Check sheet for the modelled part. Datum: model origin and axes. Units: mm. Face numbers are marked on the shaded views. A direction names the side the tool comes from. Coordinates: 2 decimals unless noted, no trailing zeros. Order: outer loops, then holes, each group sorted by start corner. A loop starts at its lowest first (then second) coordinate and runs counter-clockwise, first axis right, second up.
1. Set-up check for the marked faces 1, 2 and 3: record each of +Z, -Z, +X, -X, +Y, -Y from which the full face is reachable in a straight line by a thin tool's end or side.
2. Cross-section at A-A (y = 0). Enter the section's corners in (x, z), then the cut area to 3 significant figures.
3. Gauge pin test, flat ends, axial feed: pin 1 Ø16 at (y, z) = (5.5, 36.5) entering from +X; pin 2 Ø6.5 at (y, z) = (0, 13.5) entering from +X; pin 3 Ø3 at (y, z) = (-0.5, 14.5) entering from +X; pin 4 Ø4 at (x, y) = (18.5, -11.5) entering from -Z. Record the tip position at first contact, or that the pin passes through.
4. Cross-section at B-B (x = 11.25). Enter the section's corners in (y, z), then the cut area to 3 significant figures.
5. Draft check along Z on the marked faces 4, 5, 6 and 7. Enter one of: released by +Z, released by -Z, zero draft, split by the parting line, or undercut.
6. Thickness scan on line 1 (Y direction, x = 0.45, z = 36.5); line 2 (Y direction, x = -0.85, z = 36.5); line 3 (X direction, y = -7, z = 4). Record the ranges inside material, lowest first.
7. Cross-section at D-D (x = 3). Enter the section's corners in (y, z), then the cut area to 3 significant figures.
8. Cross-section at C-C (z = 13.5). Enter the section's corners in (x, y), then the cut area to 4 significant figures.
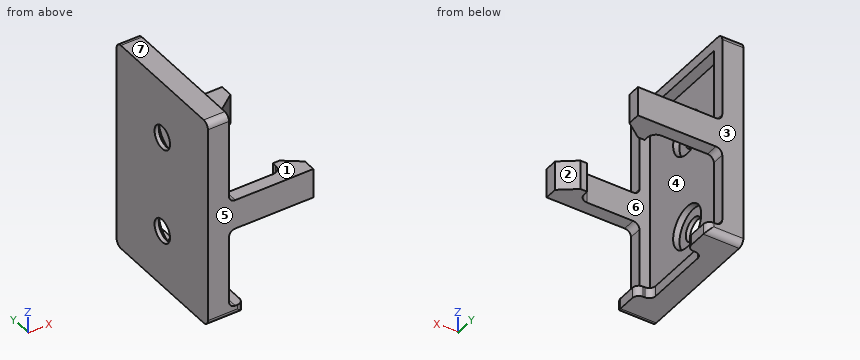
```python
from build123d import *

# Parameters (mm, degrees)
SKETCH1_W           = 2.5
SKETCH1_H           = 32.5
BOSS_EXTRUDE1_DEPTH = 50
SKETCH5_R           = 2.75
CUT_EXTRUDE5_DEPTH  = 30.5
SKETCH6_R           = 5
CUT_EXTRUDE6_DEPTH  = 1.5
SKETCH7_W           = 50
SKETCH7_H           = 32.5
SKETCH7_W_2         = 45
SKETCH7_H_2         = 26.5
BOSS_EXTRUDE2_DEPTH = 2.5
SKETCH8_W           = 7
SKETCH8_H           = 6
BOSS_EXTRUDE3_DEPTH = 20
CUT_EXTRUDE9_DEPTH  = 20
SKETCH10_W          = 3.5
SKETCH10_H          = 7.25
BOSS_EXTRUDE4_DEPTH = 2.5
FILLET1_R           = 1.5


with BuildPart() as part:
    # Sketch1 → Boss-Extrude1 (new body)
    with BuildSketch(Plane.XY):
        Rectangle(SKETCH1_W, SKETCH1_H)
    extrude(amount=BOSS_EXTRUDE1_DEPTH)

    # Sketch5 → Cut-Extrude5 (cut)
    with BuildSketch(Plane.ZY.offset(1.25)):
        with Locations((13.5, 0)):
            Circle(SKETCH5_R)
        with Locations((36.5, 0)):
            Circle(SKETCH5_R)
    extrude(amount=-CUT_EXTRUDE5_DEPTH, mode=Mode.SUBTRACT)

    # Sketch6 → Cut-Extrude6 (cut)
    with BuildSketch(Plane(origin=(1.25, 0, 0), x_dir=(0, 0, -1), z_dir=(1, 0, 0))):
        with Locations((-36.5, 0)):
            Circle(SKETCH6_R)
        with Locations((-13.5, 0)):
            Circle(SKETCH6_R)
    extrude(amount=-CUT_EXTRUDE6_DEPTH, mode=Mode.SUBTRACT)

    # Sketch7 → Boss-Extrude2 (add)
    with BuildSketch(Plane(origin=(1.25, 0, 0), x_dir=(0, 0, -1), z_dir=(1, 0, 0))):
        with Locations((-25, 0)):
            Rectangle(SKETCH7_W, SKETCH7_H)
        with Locations((-25, 0)):
            Rectangle(SKETCH7_W_2, SKETCH7_H_2, mode=Mode.SUBTRACT)
    extrude(amount=BOSS_EXTRUDE2_DEPTH)

    # Sketch8 → Boss-Extrude3 (add)
    with BuildSketch(Plane(origin=(3.75, 0, 0), x_dir=(0, 0, -1), z_dir=(1, 0, 0))):
        with Locations((-25, 13.25)):
            Rectangle(SKETCH8_W, SKETCH8_H)
        with Locations((-25, -13.25)):
            Rectangle(SKETCH8_W, SKETCH8_H)
    extrude(amount=BOSS_EXTRUDE3_DEPTH)

    # Sketch9 → Cut-Extrude9 (cut)
    with BuildSketch(Plane(origin=(0, 0, 21.5), x_dir=(-1, 0, 0), z_dir=(0, 0, -1))):
        with BuildLine():
            Line((-3.75, 13.25), (-16.15, 13.25))
            ThreePointArc((-16.15, 13.25), (-17.564213562, 12.664213562), (-18.15, 11.25))
            Line((-18.15, 11.25), (-18.15, 10.25))
            Line((-18.15, 10.25), (-3.75, 10.25))
            Line((-3.75, 10.25), (-3.75, 13.25))
        make_face()
        with BuildLine():
            Line((-3.75, -10.25), (-3.75, -13.25))
            Line((-3.75, -13.25), (-16.15, -13.25))
            ThreePointArc((-16.15, -13.25), (-17.564213562, -12.664213562), (-18.15, -11.25))
            Line((-18.15, -11.25), (-18.15, -10.25))
            Line((-18.15, -10.25), (-3.75, -10.25))
        make_face()
        Polygon((-23.75, 13.25), (-19.75, 10.25), (-23.75, 10.25), align=None)
        Polygon((-23.75, -10.25), (-23.75, -13.25), (-19.75, -10.25), align=None)
    extrude(amount=-CUT_EXTRUDE9_DEPTH, mode=Mode.SUBTRACT)

    # Sketch10 → Boss-Extrude4 (add)
    with BuildSketch(Plane.XY.offset(2.5)):
        with Locations((5.5, -12.625)):
            Rectangle(SKETCH10_W, SKETCH10_H)
        with Locations((5.5, 12.625)):
            Rectangle(SKETCH10_W, SKETCH10_H)
    extrude(amount=-BOSS_EXTRUDE4_DEPTH)

    # Fillet1
    fillet1_edges = [part.edges().sort_by_distance(p)[0] for p in [
        (3, -16.25, 0),
        (3, 16.25, 0),
        (1.25, 16.25, 50),
        (1.25, -16.25, 50),
        (3.75, -14.75, 28.5),
        (3.75, 14.75, 28.5),
        (3.75, 14.75, 21.5),
        (3.75, -14.75, 21.5),
        (7.25, -16.25, 1.25),
        (3.75, -14.75, 2.5),
        (3.75, 14.75, 2.5),
        (7.25, 16.25, 1.25),
        (7.25, -9, 1.25),
        (3.75, -9, 1.25),
        (7.25, 9, 1.25),
        (3.75, 9, 1.25),
    ]]
    fillet(fillet1_edges, radius=FILLET1_R)


solid = part.part
```
Data:
1. face 1: +Z, +X, +Y, -Y
1. face 2: +Z, -Z, +X
1. face 3: +Z, -Z, +X, -X, +Y
2. outline: (-1.25, 0) - (3.75, 0) - (3.75, 2.5) - (1.25, 2.5) - (1.25, 8.5) - (-0.25, 8.5) - (-0.25, 10.75) - (-1.25, 10.75) - close; (-1.25, 16.25) - (-0.25, 16.25) - (-0.25, 18.5) - (1.25, 18.5) - (1.25, 31.5) - (-0.25, 31.5) - (-0.25, 33.75) - (-1.25, 33.75) - close; (-1.25, 39.25) - (-0.25, 39.25) - (-0.25, 41.5) - (1.25, 41.5) - (1.25, 47.5) - (3.75, 47.5) - (3.75, 50) - (-1.25, 50) - close
2. area: 96.5 mm2
3. pin 1: stops at x = 3.75
3. pin 2: stops at x = -0.25
3. pin 3: passes through
3. pin 4: stops at z = 21.5
4. outline: (-16.25, 21.5) - (-13.25, 21.5) - (-13.25, 28.5) - (-16.25, 28.5) - close; (13.25, 21.5) - (16.25, 21.5) - (16.25, 28.5) - (13.25, 28.5) - close
4. area: 42.0 mm2
5. face 4: undercut
5. face 5: zero draft
5. face 6: undercut
5. face 7: released by +Z
6. line 1: y = -16.25 to -5, 5 to 16.25
6. line 2: y = -16.25 to -2.75, 2.75 to 16.25
6. line 3: x = -1.25 to 1.25
7. outline: (-16.25, 1.5) arc R1.5 ccw to (-14.75, 0) - (14.75, 0) arc R1.5 ccw to (16.25, 1.5) - (16.25, 48.5) arc R1.5 ccw to (14.75, 50) - (-14.75, 50) arc R1.5 ccw to (-16.25, 48.5) - close; hole (-13.25, 2.5) - (13.25, 2.5) - (13.25, 47.5) - (-13.25, 47.5) - close
7. area: 431 mm2
8. outline: (-1.25, -16.25) - (3.75, -16.25) - (3.75, -13.25) - (1.25, -13.25) - (1.25, -5) - (-0.25, -5) - (-0.25, -2.75) - (-1.25, -2.75) - close; (-1.25, 2.75) - (-0.25, 2.75) - (-0.25, 5) - (1.25, 5) - (1.25, 13.25) - (3.75, 13.25) - (3.75, 16.25) - (-1.25, 16.25) - close
8. area: 75.75 mm2
